Could you check a few things on this model? Use its own coordinates, in mm. Give positions to 0.01 mm unless a question says otherwise; leave off trailing zeros. Loops run counter-clockwise (first coordinate to the right, second up) from the corner with the lowest first, then second, coordinate; pieces in that order, holes last. Notation, with made-up numbers: (-25, -37) - (33, -37) arc R17 cw to (33, -17) - close; hole circle Ø7 at (15, -26). An arc over 180 degrees is marked (long way). Write each question's results on one line, items separated by ' | '. Start each with the question number.
1) I want a section at D-D, the plane x = 15. Write out the boundary of the cut face in (y, z), and give its area (3 significant figures).
2) I want a section at B-B, the plane y = 0.5. Write out the boundary of the cut face in (x, z), and give its area (3 significant figures).
3) I want a section at C-C, the plane z = -15.75. Write out the boundary of the cut face in (x, y), and give its area (3 significant figures).
4) If I drill on probe 1 along Z at (x, y) = (36.5, 0.5); probe 2 along X at (y, z) = (0.45, -14.5); probe 3 along X at (y, z) = (0.85, -14), over which ranges is the centre line in solid material (lowest first)? Write a range as [from, to].
5) I'm going to push a flat-ended pin straight in: pin 1 (8 mm diameter, centred on x = 41.5, z = -16, fed in from +Y). Where does the tip first touch, or does it pass through?
6) I want a section at A-A, the plane x = 34. Write out the boundary of the cut face in (y, z), and give its area (3 significant figures).
7) If we mould it in two halves opening along Z, with no side actions, what happens to faces 1 (the face through (13.5, 0.5, -15.7)), 2 (the face through (35, 0, -12))? For each: +Z half, -Z half, draft (parallel to the pull), parting line (faces both ways), or undercut.
from build123d import *

# Parameters (mm, degrees)
BOSS_EXTRUDE1_DEPTH = 1


with BuildPart() as part:
    # Sketch1 → Boss-Extrude1 (new body)
    with BuildSketch(Plane(origin=(0, 0, 0), x_dir=(1, 0, 0), z_dir=(0, 1, 0))):
        with BuildLine():
            Line((0, 31.5), (0, 0))
            Line((0, 0), (71.25, 0))
            Line((71.25, 0), (71.25, 12.5))
            Line((71.25, 12.5), (16.75, 12.5))
            ThreePointArc((16.75, 12.5), (13.5, 15.75), (16.75, 19))
            Line((16.75, 19), (71.25, 19))
            Line((71.25, 19), (71.25, 31.5))
            Line((71.25, 31.5), (0, 31.5))
        make_face()
    extrude(amount=BOSS_EXTRUDE1_DEPTH)


solid = part.part
Answers:
1) outline: (0, -31.5) - (1, -31.5) - (1, -18.49) - (0, -18.49) - close; (0, -13.01) - (1, -13.01) - (1, 0) - (0, 0) - close | area: 26.0 mm2
2) outline: (0, -31.5) - (71.25, -31.5) - (71.25, -19) - (16.75, -19) arc R3.25 cw to (16.75, -12.5) - (71.25, -12.5) - (71.25, 0) - (0, 0) - close | area: 1,870 mm2
3) outline: (0, 0) - (13.5, 0) - (13.5, 1) - (0, 1) - close | area: 13.5 mm2
4) probe 1: z = [-31.5, -19], [-12.5, 0] | probe 2: x = [0, 13.75] | probe 3: x = [0, 14.01]
5) pin 1: stops at y = 1
6) outline: (0, -31.5) - (1, -31.5) - (1, -19) - (0, -19) - close; (0, -12.5) - (1, -12.5) - (1, 0) - (0, 0) - close | area: 25.0 mm2
7) face 1: undercut | face 2: draft
